Read the model definition and answer for the solid it produces. Units are mm, in the model's axes. Face numbers are marked on the shaded views. Give positions to 0.01 mm unless a question says otherwise; leave off trailing zeros. Write each loop counter-clockwise with the first axis right and the second up, starting at its lowest first coordinate (ties: lowest second). Pieces come first, ordered by that corner, then holes. Notation, with made-up numbers: (87, -36) -> (101, -36) arc R14 ccw to (101, -21) -> close; hole circle Ø1 at (-30.75, -16.75). An arc over 180 degrees is marked (long way). Write item = value, one per line.
from build123d import *

# Parameters (mm, degrees)
F0_R     = 50.8
F1_DEPTH = 15.875
F2_R     = 44.45
F3_DEPTH = 15.876
F4_R     = 3.17499


# Not quite as in the source:
# - a fillet or chamfer is up to 0.001 mm smaller than in the source, because OpenCascade refuses the exact size


with BuildPart() as f1:
    # F0 (on Front) → F1 (new body)
    with BuildSketch(Plane.XZ):
        Circle(F0_R)
    extrude(amount=F1_DEPTH)

    # F2 (on Front) → F3 (cut, through all)
    with BuildSketch(Plane.XZ):
        Circle(F2_R)
    extrude(amount=F3_DEPTH, mode=Mode.SUBTRACT)

    # F4 (radius 3.175 in the source; OpenCascade refuses exactly that, so slightly less here)
    f4_edges = [f1.edges().sort_by_distance(p)[0] for p in [
        (-50.8, -15.875, 0),
        (-44.45, -15.875, 0),
    ]]
    fillet(f4_edges, radius=F4_R)


solid = f1.part
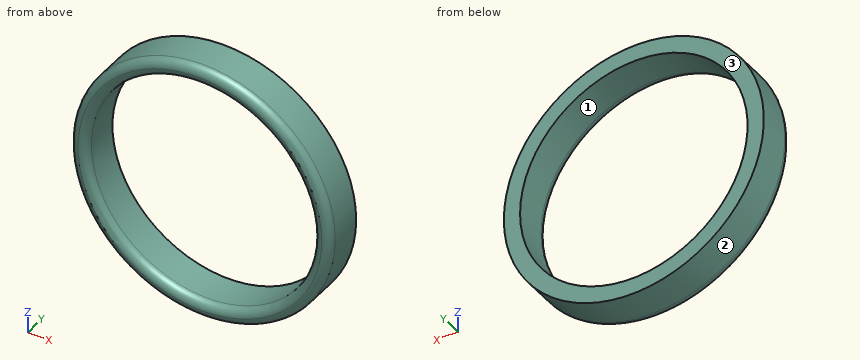
(1) The part is cut by section C-C on y = -4. Determine the outline of the cut face in (x, z).
Checks:
outline = circle Ø101.6 at (0, 0); hole circle Ø88.9 at (0, 0)
(2) For a pull along X with two mould halves and no side action, classify the marked faces 1, 2 and 3 as released by +X, released by -X, zero draft, split by the parting line, or undercut.
Checks:
face_1 = undercut
face_2 = split by the parting line
face_3 = zero draft
(3) Consider L1, parallel to Z at x = 0, y = -5.75; L2, parallel to X at y = -4.5, z = 27; L3, parallel to Z at x = -24, y = -7.5. Determine where each line is inside the solid, lowest interval first.
Checks:
L1 = -50.8 to -44.45, 44.45 to 50.8
L2 = -43.03 to -35.31, 35.31 to 43.03
L3 = -44.77 to -37.41, 37.41 to 44.77
(4) Given P1, Ø8, axis at y = -11, z = -27, coming from the -X side; P2, Ø2, axis at y = -4, z = -12.5, coming from the +X side; P3, Ø3, axis at y = -13.5, z = 13, coming from the -X side, each flat-ended and moving along its own axis, determine where each tip first touches the part or whether it passes through.
Checks:
P1 = -45.3
P2 = 49.48
P3 = -49.45
